from build123d import *

# Parameters (mm, degrees)
SKETCH1_R           = 14
BOSS_EXTRUDE1_DEPTH = 53.34
SKETCH2_R           = 2.4
SKETCH2_R_2         = 1.27
BOSS_EXTRUDE2_DEPTH = 6


with BuildPart() as part:
    # Sketch1 → Boss-Extrude1 (new body)
    with BuildSketch(Plane(origin=(0, 0, 0), x_dir=(1, 0, 0), z_dir=(0, 1, 0))):
        with Locations(Location((0, 0, 0), (0, 0, 270))):
            Circle(SKETCH1_R)
    extrude(amount=BOSS_EXTRUDE1_DEPTH)

    # Sketch2 → Boss-Extrude2 (add)
    with BuildSketch(Plane(origin=(0, 53.34, 0), x_dir=(1, 0, 0), z_dir=(0, 1, 0))):
        with Locations(Location((0, 0, 0), (0, 0, 270))):
            Circle(SKETCH2_R)
        with Locations(Location((8, 0, 0), (0, 0, 270))):
            Circle(SKETCH2_R_2)
        with Locations(Location((0, -8, 0), (0, 0, 270))):
            Circle(SKETCH2_R_2)
        with Locations(Location((-8, 0, 0), (0, 0, 270))):
            Circle(SKETCH2_R_2)
        with Locations(Location((0, 8, 0), (0, 0, 270))):
            Circle(SKETCH2_R_2)
    extrude(amount=BOSS_EXTRUDE2_DEPTH)


solid = part.part
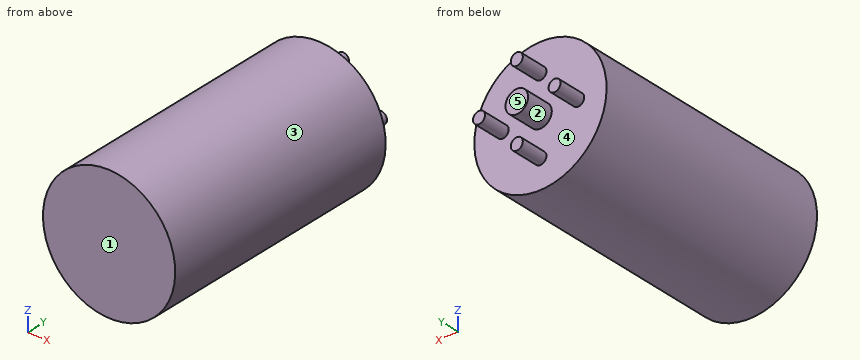
Could you check a few things on this model? Use its own coordinates, in mm. Face numbers are marked on the shaded views. A direction names the side the tool comes from. Give positions to 0.01 mm unless a question says otherwise; leave off trailing zeros. Write each loop counter-clockwise with the first axis right and the second up, starting at its lowest first coordinate (ties: lowest second). Pieces come first, ordered by that corner, then holes. Notation, with made-up numbers: (-22.5, -25) -> (18.5, -25) arc R25 ccw to (18.5, 14) -> close; hole circle Ø3 at (84, 31.5). An arc over 180 degrees is marked (long way). Write each question's results on one line, items separated by ' | '. Start each with the question number.
Q1. Suppose I cut it at A-A, the plane x = 0. List the corners of the cut face in (y, z) for me, and give its area (3 significant figures).
Q2. Suppose I cut it at B-B, the plane z = 8. List the corners of the cut face in (x, y) for me.
Q3. I need wall thicknesses on probe 1 along Y at (x, z) = (3, -8); probe 2 along X at (y, z) = (42, 0); probe 3 along Z at (x, y) = (-10.5, 4.5). Which ranges of each line are inside material? Lowest first, please.
Q4. Which directions (+Z, -Z, +X, -X, +Y, -Y) give clear straight access to the entire face, cutting with the end or side of a thin tool? Please do the marked faces 4 and 5.
Q5. I'm going to push flat-ended pins straight in: pin 1 Ø6 at (x, y) = (2.5, 51.5) entering from -Z; pin 2 Ø6 at (x, y) = (9.5, 49.5) entering from +Z; pin 3 Ø6 at (x, z) = (7.5, -9) entering from +Y; pin 4 Ø8 at (x, y) = (6, 24) entering from -Z. Where does each tip first touch, or does it pass through?
Q6. Suppose I cut it at D-D, the plane x = 8. List the corners of the cut face in (y, z) for me, and give its area (3 significant figures).
Q7. We'd pull the mould along Z, two halves only. Please class the marked faces 1, 2 and 3: +Z half, -Z half, draft (parallel to the pull), parting line (faces both ways), or undercut.
Q8. Suppose I cut it at C-C, the plane y = 25. List the corners of the cut face in (x, z) for me.
Outcome:
1) outline: (0, -14) -> (53.34, -14) -> (53.34, -9.27) -> (59.34, -9.27) -> (59.34, -6.73) -> (53.34, -6.73) -> (53.34, -2.4) -> (59.34, -2.4) -> (59.34, 2.4) -> (53.34, 2.4) -> (53.34, 6.73) -> (59.34, 6.73) -> (59.34, 9.27) -> (53.34, 9.27) -> (53.34, 14) -> (0, 14) -> close | area: 1,550 mm2
2) outline: (-11.49, 0) -> (11.49, 0) -> (11.49, 53.34) -> (1.27, 53.34) -> (1.27, 59.34) -> (-1.27, 59.34) -> (-1.27, 53.34) -> (-11.49, 53.34) -> close
3) probe 1: 0 to 53.34 | probe 2: -14 to 14 | probe 3: -9.26 to 9.26
4) face 4: +Y | face 5: +Z, -Z, +X, -X, +Y
5) pin 1: z = -14 | pin 2: z = 12.4 | pin 3: y = 53.34 | pin 4: z = -13.86
6) outline: (0, -11.49) -> (53.34, -11.49) -> (53.34, -1.27) -> (59.34, -1.27) -> (59.34, 1.27) -> (53.34, 1.27) -> (53.34, 11.49) -> (0, 11.49) -> close | area: 1,240 mm2
7) face 1: draft | face 2: undercut | face 3: parting line
8) outline: circle Ø28 at (0, 0)
